The listing builds one solid part. Answer for the finished solid, in the listing's coordinates (mm). A direction names the side the tool comes from. Round coordinates to 2 decimals unless told otherwise and drop trailing zeros.
Item 1: A tool of negligible diameter and unlimited length cuts with its end or side. For faces 1 (the face through (19.058, 57.008, -2.24)), 2 (the face through (-6, -112, 3)), 3 (the face through (-4.3, -112.1, -1.5)), from which of +Z, -Z, +X, -X, +Y, -Y can it reach the whole face along a straight path? Write none if from no direction.
Item 2: Each of these flat-tipped pins is pushed along its axis until it touches: pin 1 (25 mm diameter, centred on x = 13.5, y = -140, fed in from +Z); pin 2 (3 mm diameter, centred on x = 20.5, z = 1.5, fed in from -Y); pin 3 (1.5 mm diameter, centred on y = -104.5, z = 0.5, fed in from -X); pin 4 (3 mm diameter, centred on x = 0, z = -2.5, fed in from +Y). Where does it stop, or does it pass through?
Item 3: Find the intervals of material crossed by probe 1 along X at (y, z) = (-123.5, 0); probe 2 along Y at (x, z) = (2.5, -2.5); probe 3 along Z at (x, y) = (-6, -20.5), in increasing order.
Item 4: For a pull along X with two mould halves and no side action, classify faces 4 (the face through (44, -112, -4.3)), 5 (the face through (18.04, -290.12, 2.24)), 6 (the face through (-5, -112, -3)) as +X half, -X half, draft (parallel to the pull), parting line (faces both ways), or undercut.
Autodesk Inventor part; units mm, degrees
ref_plane "Work Plane2" through (18.5, 35, 0) normal (-1, 0, 0) x (0, 0, 1)
ref_plane "Work Plane3" through (17.5, -260.9983, 0) normal (0.309017, 0.9510565, 0) x (0, 0, 1)
ref_plane "Section Plane" through (-7.0697, 35.0864, 0) normal (-0.0033784, -0.9999943, 0) x (0, 0, 1)
ref_plane "Work Plane2" through (18.5, 35, 0) normal (-1, 0, 0) x (0, 0, 1)
ref_plane "Work Plane3" through (17.5, -260.9983, 0) normal (0.309017, 0.9510565, 0) x (0, 0, 1)
sketch "Path" plane through (0, 0, 0) normal (0, 0, 1) x (1, 0, 0)
  arc A0 (44.0697, 34.9136) -> (-7.0697, 35.0864) centre (18.5, 35) ccw
  arc A1 (-8.0697, -260.9119) -> (43.0697, -261.0847) centre (17.5, -260.9983) ccw
  line L0 (-8.0697, -260.9119) -> (-7.0697, 35.0864)
  line L1 (44.0697, 34.9136) -> (43.0697, -261.0847)
ref_plane "Section Plane" through (-7.0697, 35.0864, 0) normal (-0.0033784, -0.9999943, 0) x (0, 0, 1)
sketch "Section Sketch" plane through (-7.0697, 35.0864, 0) normal (-0.0033784, -0.9999943, 0) x (0, 0, 1)
  line L0 (-4.3, -1.155) -> (4.3, -1.155)
  line L1 (4.3, -1.155) -> (4.3, 1.155)
  line L2 (4.3, 1.155) -> (-4.3, 1.155)
  line L3 (-4.3, 1.155) -> (-4.3, -1.155)
  line L4 (-1.5, -2.5) -> (1.5, -2.5)
  line L5 (1.5, -2.5) -> (1.5, 2.5)
  line L6 (1.5, 2.5) -> (-1.5, 2.5)
  line L7 (-1.5, 2.5) -> (-1.5, -2.5)
  line L8 (-1.5, 0) -> (1.5, 0) construction
  line L9 (-3, -3.555) -> (-1.5, -3.555)
  line L10 (-1.5, -3.555) -> (-1.5, 3.555)
  line L11 (-1.5, 3.555) -> (-3, 3.555)
  line L12 (-3, 3.555) -> (-3, -3.555)
  line L13 (1.5, -3.555) -> (3, -3.555)
  line L14 (3, -3.555) -> (3, 3.555)
  line L15 (3, 3.555) -> (1.5, 3.555)
  line L16 (1.5, 3.555) -> (1.5, -3.555)
  line L17 (-4.3, 0) -> (4.3, 0) construction
  point P0 (0, 0)
  point P1 (0, 0)
  dimension "d21" = 2.31
  dimension "d22" = 5
  dimension "d23" = 3
  dimension "d24" = 1.5
  dimension "d31" = 7.11
  dimension "d32" = 8.6
sweep "Solid" add profiles "Section Sketch" path "Path"
pattern_of_one "Strand Pattern"
equation "\"d21\" = da_d2"
equation "\"d22\" = da_d1"
equation "\"d23\" = da_b1"
equation "\"d24\" = da_t1 + da_t2"
equation "\"d30\" = da_pt"
equation "\"da_p\" = 8"
equation "\"da_b1\" = 3"
equation "\"da_h2\" = 7.11"
equation "\"da_h3\" = 7.11"
equation "\"da_d1\" = 5"
equation "\"da_d2\" = 2.31"
equation "\"da_pt\" = 5.64"
equation "\"da_b\" = 8.6"
equation "\"da_t1\" = 0.75"
equation "\"da_t2\" = 0.75"
properties part number "Roller Chain"
Check values:
1. face 1: +Z, -Z
1. face 2: +Z
1. face 3: none
2. pin 1: passes through
2. pin 2: stops at y = -290.08
2. pin 3: stops at x = -10.04
2. pin 4: stops at y = 58.65
3. probe 1: x = -10.11 to -5.11, 41.03 to 46.03
3. probe 2: y = -285.96 to -277.11, 50.12 to 59.34
3. probe 3: z = -3 to 3
4. face 4: draft
4. face 5: parting line
4. face 6: undercut
